Source: three-view drawing plus pictorial views. Frame: mm from the lowest corner of the part. A direction names the side the tool comes from. Coordinates: 2 decimals unless noted, no trailing zeros. Loops run counter-clockwise (first coordinate to the right, second up) from the corner with the lowest first, then second, coordinate; pieces in that order, holes last. Notation, with made-up numbers: M 55.5,-30.5 L 88.5,-30.5 A24 cw 88.5,2.5 Z; hole C -10,-15 d4. An arc over 180 degrees is marked long. Use a Markdown table: item, result. Add a question column.
1. Section A-A on x = 14. Output: boundary loops of the cut face in (y, z).
2. Draft query along Y for the marked faces 1, 2 and 3. Return one class per face: +Y half, -Y half, draft (parallel to the pull), parting line (faces both ways), or undercut.
3. Set-up query: the marked faces 4, 5 and 6. Return all of +Z, -Z, +X, -X, +Y, -Y with unobstructed straight access to the full face (end or side cutting, diameter ignored); none if empty.
4. Pin query (flat end, axial travel): pin 1 (1 mm diameter, centred on x = 10.5, y = 5.5, fed in from +Z); pin 2 (4 mm diameter, centred on x = 19.75, y = 23.96, fed in from -Z); pin 3 (5 mm diameter, centred on y = 14, z = 8, fed in from +X); pin 4 (4 mm diameter, centred on x = 5.5, z = 14.5, fed in from -Y). Return the tip coordinate at first contact, or that it passes through.
5. Section B-B on y = 14. Output: boundary loops of the cut face in (x, z), then the cut area to 3 significant figures.
6. Line query: L1, parallel to Y at x = 19.75, z = 2.1 (1 decimal); L2, parallel to Y at x = 14, z = 4.75; L3, parallel to Z at x = 2.75, y = 20. Output: solid intervals per line, ascending. Write a range as [from, to].
7. Section D-D on z = 4.75. Output: boundary loops of the cut face in (x, y), then the cut area to 3 significant figures.
8. Section C-C on x = 19.5. Output: boundary loops of the cut face in (y, z) (1 decimal).
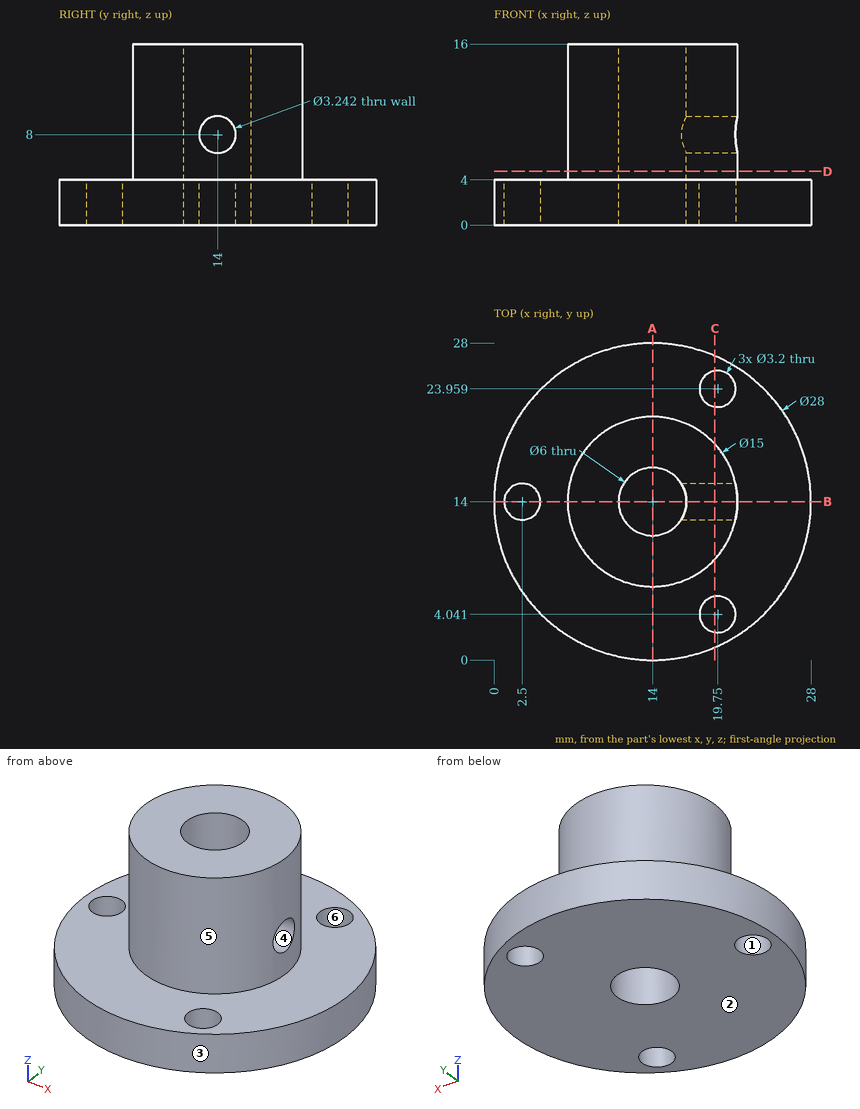
Answers below:
| question | item | result |
|---|---|---|
| 1 | outline | M 0,0 L 11,0 L 11,16 L 6.5,16 L 6.5,4 L 0,4 Z; M 17,0 L 28,0 L 28,4 L 21.5,4 L 21.5,16 L 17,16 Z |
| 2 | face 1 | undercut |
| 2 | face 2 | draft |
| 2 | face 3 | parting line |
| 3 | face 4 | +X |
| 3 | face 5 | +Z |
| 3 | face 6 | +Z, -Z |
| 4 | pin 1 | stops at z = 4 |
| 4 | pin 2 | stops at z = 0 |
| 4 | pin 3 | stops at x = 21.5 |
| 4 | pin 4 | stops at y = 10.26 |
| 5 | outline | M 0,0 L 0.9,0 L 0.9,4 L 0,4 Z; M 4.1,0 L 11,0 L 11,16 L 6.5,16 L 6.5,4 L 4.1,4 Z; M 17,0 L 28,0 L 28,4 L 21.5,4 L 21.5,6.38 L 17,6.38 Z; M 17,9.62 L 21.5,9.62 L 21.5,16 L 17,16 Z |
| 5 | area | 169 mm² |
| 6 | L1 | y = [1.2, 2.4], [5.6, 22.4], [25.6, 26.8] |
| 6 | L2 | y = [6.5, 11], [17, 21.5] |
| 6 | L3 | z = [0, 4] |
| 7 | outline | C 14,14 d15; hole C 14,14 d6 |
| 7 | area | 148 mm² |
| 8 | outline | M 1.1,0 L 2.5,0 L 2.5,4 L 1.1,4 Z; M 5.6,0 L 22.4,0 L 22.4,4 L 19.1,4 L 19.1,16 L 8.9,16 L 8.9,4 L 5.6,4 Z; M 25.5,0 L 26.9,0 L 26.9,4 L 25.5,4 Z; hole C 14,8 d3.2 |
